Geometry: final body of the model. Coordinates: model frame, mm. A direction names the side the tool comes from. Give positions to 0.01 mm unless a question says otherwise; leave off trailing zeros. Loops run counter-clockwise (first coordinate to the right, second up) from the corner with the lowest first, then second, coordinate; pieces in that order, holes last.
Autodesk Inventor part; units mm, degrees
ref_plane "Work Plane1" through (-26, 27.7, 10) normal (0, -1, 0) x (1, 0, 0)
ref_plane "Work Plane3" through (19.5, 27.7, -10) normal (0, -1, 0) x (1, 0, 0)
ref_plane "Work Plane5" through (-19.5, 27.7, 10) normal (0, 0, 1) x (1, 0, 0)
ref_plane "Work Plane1" through (-26, 27.7, 10) normal (0, -1, 0) x (1, 0, 0)
sketch "Sketch1" plane through (-26, 27.7, 10) normal (0, -1, 0) x (1, 0, 0)
  line L0 (6, -0.5) -> (6, 0)
  line L1 (0, 0) -> (6.5, 0)
  line L2 (6, 0) -> (0, 0)
  line L3 (0, 0) -> (-2, 0)
  arc A0 (0, 0) -> (-2, -2) centre (0, -2) ccw
  line L4 (-2, 0) -> (-2, 0)
  line L5 (0, 0) -> (-2, 0)
  line L6 (-2, -2) -> (-2, -3.75)
  line L7 (-2, -2) -> (-2, 0)
  arc A1 (0, 0) -> (-2, -2) centre (0, -2) ccw
  line L8 (0, 0) -> (-2, 0)
  arc A2 (-2, -18) -> (0, -20) centre (0, -18) ccw
  line L9 (-2, -2) -> (-2, -18)
  line L10 (-2, -18) -> (-2, -20)
  line L11 (-2, -20) -> (0, -20)
  line L12 (0, -20) -> (6.5, -20)
  line L13 (6, -19.5) -> (6, -20)
  line L14 (6, -19.5) -> (6, -0.5)
  point P0 (26, -10)
extrude "Extrusion1" add sketch "Sketch1" along normal blind 10
ref_plane "Work Plane3" through (19.5, 27.7, -10) normal (0, -1, 0) x (1, 0, 0)
sketch "Sketch2" plane through (19.5, 27.7, -10) normal (0, -1, 0) x (1, 0, 0)
  line L0 (0.5, 19.5) -> (0.5, 0.5)
  line L1 (0.5, 19.5) -> (0.5, 20)
  line L2 (0, 20) -> (6.5, 20)
  line L3 (0.5, 0.4979) -> (0.5, -0.0021)
  arc A0 (6.5, 0) -> (8.5, 2) centre (6.5, 2) ccw
  line L4 (0, 0) -> (6.5, 0)
  line L5 (8.5, 2) -> (6.5, 2)
  line L6 (6.5, 2) -> (6.5, 0)
  line L7 (6.5, 0) -> (8.5, 0)
  line L8 (8.5, 0) -> (8.5, 2)
  line L9 (0.5, 20) -> (8.5, 20)
  line L10 (8.5, 20) -> (8.5, 0)
  line L11 (8.5, 0) -> (0.5, 0)
  line L12 (0.5, 0) -> (0.5, 20)
  point P0 (-19.5, 10)
  point P1 (0.5, 0.5)
  dimension "d4" = 0.5
extrude "Extrusion2" add sketch "Sketch2" along normal blind 10
ref_plane "Work Plane5" through (-19.5, 27.7, 10) normal (0, 0, 1) x (1, 0, 0)
sketch "Sketch3" plane through (-19.5, 27.7, 10) normal (0, 0, 1) x (1, 0, 0)
  line L0 (-8.5, 0) -> (-8.5, -10)
  line L1 (47.5, 0) -> (47.5, 2.5)
  line L2 (-8.5, -10) -> (47.5, -10)
  line L3 (47.5, -10) -> (47.5, 2.5)
  line L4 (47.5, 2.5) -> (-8.5, 2.5)
  line L5 (-8.5, 2.5) -> (-8.5, -10)
  point P0 (19.5, -27.7)
extrude "Extrusion3" add sketch "Sketch3" along normal blind 10
ref_plane "Work Plane4" through (19.5, 27.7, -10) normal (0, 1, 0) x (1, 0, 0)
sketch "Sketch4" plane through (19.5, 27.7, -10) normal (0, 1, 0) x (1, 0, 0)
  arc A0 (6.415, -13.3929) -> (6.415, -16.6071) centre (4.5, -15) ccw
  circle A1 centre (4.5, -15) radius 2.5
  arc A2 (6.415, -3.3929) -> (6.415, -6.6071) centre (4.5, -5) ccw
  circle A3 centre (4.5, -5) radius 2.5
  arc A4 (-45.415, -16.6071) -> (-45.415, -13.3929) centre (-43.5, -15) ccw
  circle A5 centre (-43.5, -15) radius 2.5
  arc A6 (-45.415, -6.6071) -> (-45.415, -3.3929) centre (-43.5, -5) ccw
  circle A7 centre (-43.5, -5) radius 2.5
  point P0 (-19.5, -10)
  point P1 (6.415, -3.3929)
  point P2 (6.415, -13.3929)
  point P3 (-45.415, -16.6071)
  point P4 (-45.415, -6.6071)
extrude "Extrusion4" cut sketch "Sketch4" against normal blind 10
ref_plane "Work Plane6" through (-28, 30.2, -3.75) normal (-1, 0, 0) x (0, 0, 1)
sketch "Sketch5" plane through (-28, 30.2, -3.75) normal (-1, 0, 0) x (0, 0, 1)
  line L0 (-6.25, -12.5) -> (23.75, -12.5)
  line L1 (-6.25, -2.5) -> (-6.25, -12.5)
  line L2 (23.75, -12.5) -> (-6.25, -12.5)
  line L3 (-6.25, -12.5) -> (-6.25, -2.5)
  line L4 (-6.25, -2.5) -> (23.75, -2.5)
  line L5 (23.75, -2.5) -> (23.75, -12.5)
  point P0 (3.75, -30.2)
extrude "Extrusion5" add sketch "Sketch5" along normal blind 11.915
ref_plane "Work Plane7" through (19.5, 27.7, -10) normal (0, 0, -1) x (-1, 0, 0)
sketch "Sketch6" plane through (19.5, 27.7, -10) normal (0, 0, -1) x (-1, 0, 0)
  line L0 (39.5, 0) -> (39.5, -10)
  line L1 (47.5, 0) -> (59.415, 0)
  line L2 (39.5, -10) -> (59.415, -10)
  line L3 (59.415, -10) -> (59.415, 0)
  line L4 (59.415, 0) -> (39.5, 0)
  line L5 (39.5, 0) -> (39.5, -10)
  point P0 (19.5, -27.7)
extrude "Extrusion6" add sketch "Sketch6" along normal blind 10
ref_plane "Work Plane8" through (-39.915, 30.2, -3.75) normal (-1, 0, 0) x (0, 0, 1)
sketch "Sketch7" plane through (-39.915, 30.2, -3.75) normal (-1, 0, 0) x (0, 0, 1)
  line L0 (-16.25, -12.5) -> (-16.25, -2.5)
  line L1 (-16.25, -12.5) -> (-6.25, -12.5)
  line L2 (-6.25, -12.5) -> (-6.25, -2.5)
  line L3 (-6.25, -2.5) -> (-16.25, -2.5)
  line L4 (-16.25, -2.5) -> (-16.25, -12.5)
  line L5 (23.75, -12.5) -> (23.75, -2.5)
  line L6 (23.75, -2.5) -> (13.75, -2.5)
  line L7 (13.75, -2.5) -> (13.75, -12.5)
  line L8 (13.75, -12.5) -> (23.75, -12.5)
  line L9 (23.75, -12.5) -> (23.75, -2.5)
  point P0 (3.75, -30.2)
  point P1 (23.75, -12.5)
  dimension "d15" = 10
  dimension "d16" = 10
extrude "Extrusion7" add sketch "Sketch7" along normal blind 20
ref_plane "Work Plane9" through (19.5, 27.7, -20) normal (0, 0, -1) x (-1, 0, 0)
sketch "Sketch9" plane through (-26, 17.7, 10) normal (0, -1, 0) x (1, 0, 0)
  line L0 (-13.915, 0) -> (-33.915, 0)
  line L1 (-13.915, 0) -> (-33.915, 0)
  line L2 (-33.915, 0) -> (-33.915, 10)
  line L3 (-33.915, 10) -> (-13.915, 10)
  line L4 (-13.915, 10) -> (-13.915, 0)
  point P0 (26, -10)
  point P1 (-33.915, 0)
extrude "Extrusion9" add sketch "Sketch9" along normal blind 20
ref_plane "Work Plane2" through (-39.915, 27.7, 15) normal (0, 0, -1) x (-1, 0, 0)
sketch "Sketch10" plane through (-39.915, 27.7, 15) normal (0, 0, -1) x (-1, 0, 0)
  line L0 (20, -30) -> (0, -30)
  line L1 (-59.915, -10) -> (-67.915, -10)
  line L2 (0, -30) -> (-59.915, -10)
  line L3 (0, -30) -> (0, -10)
  line L4 (0, -10) -> (-59.915, -10)
  point P0 (-39.915, -27.7)
extrude "Extrusion10" add sketch "Sketch10" along normal mid plane 4
ref_plane "Work Plane10" through (-19.5, 27.7, 20) normal (0, 0, 1) x (1, 0, 0)
thread "Thread1"
thread "Thread2"
thread "Thread3"
thread "Thread4"
sketch "Sketch13" plane through (-19.5, 27.7, 20) normal (0, 0, 1) x (1, 0, 0)
  line L0 (-20.415, -10) -> (-20.415, 0)
  line L1 (-20.415, 0) -> (-30.415, 0)
  line L2 (-20.415, 0) -> (-40.415, 0)
  line L3 (-30.415, 0) -> (-30.415, -5)
  line L4 (-20.415, -10) -> (-20.415, -30)
  line L5 (-20.415, -30) -> (-20.415, -20)
  line L6 (-20.415, -20) -> (-30.415, -20)
  circle A0 centre (-30.415, -5) radius 2.5
  circle A1 centre (-30.415, -20) radius 2.5
  point P0 (19.5, -27.7)
  dimension "d40" = 10
  dimension "d41" = 5
  dimension "d42" = 10
  dimension "d43" = 10
  dimension "d44" = 5
  dimension "d45" = 5
extrude "Extrusion12" cut sketch "Sketch13" against normal through all
sketch "Sketch14" plane through (-59.915, 27.7, -10) normal (0, 0, 1) x (1, 0, 0)
  line L0 (20, 0) -> (20, -10)
  line L1 (0, -10) -> (0, 0)
  line L2 (20, 0) -> (0, 0)
  line L3 (0, 0) -> (0, -10)
  line L4 (0, -10) -> (20, -10)
  line L5 (20, -10) -> (20, 0)
  point P0 (59.915, -27.7)
  point P1 (20, -10)
extrude "Extrusion13" add sketch "Sketch14" against normal blind 2
sketch "Sketch15" plane through (-39.915, 27.7, 10) normal (0, 0, -1) x (-1, 0, 0)
  line L0 (20, -30) -> (0, -30)
  line L1 (20, 0) -> (0, 0)
  line L2 (0, 0) -> (0, -30)
  line L3 (0, -30) -> (20, -30)
  line L4 (20, -30) -> (20, 0)
  point P0 (-39.915, -27.7)
extrude "Extrusion14" cut sketch "Sketch15" against normal blind 2
sketch "Sketch16" plane through (-39.915, 27.7, 12) normal (0, 0, -1) x (-1, 0, 0)
  line L0 (-11.915, 0) -> (20, 0)
  line L1 (20, -30) -> (0, -30)
  line L2 (20, 0) -> (0, 0)
  line L3 (0, 0) -> (0, -30)
  line L4 (0, -30) -> (20, -30)
  line L5 (20, -30) -> (20, 0)
  circle A0 centre (10, -20) radius 2.5
  circle A1 centre (10, -20) radius 2.5
  circle A2 centre (10, -5) radius 2.5
  circle A3 centre (10, -5) radius 2.5
  point P0 (-39.915, -27.7)
  point P1 (0, 0)
extrude "Extrusion15" add sketch "Sketch16" along normal blind 4
sketch "Sketch17" plane through (-49.915, 22.7, -12) normal (0, 0, -1) x (-1, 0, 0)
  circle A0 centre (0, 0) radius 2.5
  point P0 (-49.915, -22.7)
extrude "Extrusion16" cut sketch "Sketch17" against normal blind 4
sketch "Sketch18" plane through (-59.915, 27.7, -10) normal (0, 0, 1) x (1, 0, 0)
  line L0 (0, -10) -> (0, 0)
  line L1 (20, 0) -> (0, 0)
  line L2 (0, -10) -> (20, -10)
  line L3 (20, -10) -> (20, 0)
  line L4 (20, 0) -> (0, 0)
  line L5 (0, 0) -> (0, -10)
  point P0 (59.915, -27.7)
extrude "Extrusion17" cut sketch "Sketch18" against normal blind 2
properties part number "servo_holder" material "PET Plastic"
Item 1: Section query A-A on y = 22.7. Return loops of the section in (x, z) (3 decimals).
Values follow:
outline: (-59.915, -20) - (-52.415, -20) - (-52.415, -12) - (-59.915, -12) - close; (-59.915, 8) - (-52.415, 8) - (-52.415, 20) - (-59.915, 20) - close; (-47.415, -20) - (-20, -20) - (-20, 10) - (20, 10) - (20, -10) - (28, -10) - (28, 20) - (-47.415, 20) - (-47.415, 8) - (-39.915, 8) - (-39.915, -12) - (-47.415, -12) - close; hole circle Ø5 at (-24, -5); hole circle Ø5 at (-24, 5); hole circle Ø5 at (24, -5); hole circle Ø5 at (24, 5)
Item 2: Section query B-B on z = -5. Return loops of the section in (x, y) (3 decimals).
Values follow:
outline: (-39.915, 17.7) - (-26.5, 17.7) - (-26.5, 27.7) - (-39.915, 27.7) - close; (-21.5, 17.7) - (-20, 17.7) - (-20, 27.7) - (-21.5, 27.7) - close; (20, 17.7) - (21.5, 17.7) - (21.5, 27.7) - (20, 27.7) - close; (26.5, 17.7) - (28, 17.7) - (28, 27.7) - (26.5, 27.7) - close
Item 3: Section query C-C on x = 24. Return loops of the section in (y, z).
Values follow:
outline: (17.7, -10) - (27.7, -10) - (27.7, -7.5) - (17.7, -7.5) - close; (17.7, -2.5) - (27.7, -2.5) - (27.7, 2.5) - (17.7, 2.5) - close; (17.7, 7.5) - (27.7, 7.5) - (27.7, 10) - (30.2, 10) - (30.2, 20) - (17.7, 20) - close
Item 4: Section query D-D on z = 14. Return loops of the section in (x, y) (3 decimals).
Values follow:
outline: (-59.915, -2.3) - (-39.915, -2.3) - (20, 17.7) - (28, 17.7) - (28, 30.2) - (-28, 30.2) - (-28, 27.7) - (-59.915, 27.7) - close; hole circle Ø5 at (-49.915, 7.7); hole circle Ø5 at (-49.915, 22.7)
Item 5: Pin query (flat end, axial travel): pin 1 (5 mm diameter, centred on x = -42, y = 14, fed in from -Z); pin 2 (8 mm diameter, centred on x = -38.5, z = 6, fed in from -Y); pin 3 (4 mm diameter, centred on x = 25, y = 25, fed in from -Z); pin 4 (16 mm diameter, centred on x = -11, y = 3, fed in from -Z). Return the tip coordinate at first contact, or that it passes through.
Values follow:
pin 1: stops at z = 8
pin 2: stops at y = -2.3
pin 3: stops at z = -10
pin 4: stops at z = 13
Item 6: Draft query along X for faces 1 (the face through (28, 22, 5)), 2 (the face through (0, 24, 10)), 3 (the face through (-52.3, 23.9, -12)). Return one class per face: +X half, -X half, draft (parallel to the pull), parting line (faces both ways), or undercut.
Values follow:
face 1: +X half
face 2: undercut
face 3: draft
Item 7: Ray query, probe 1 along Z at (x, y) = (24, 24); probe 2 along X at (y, z) = (22.7, 10.15) (3 decimals); probe 3 along X at (y, z) = (21.75, -5) (3 decimals). Return the intervals inside material, ascending.
Values follow:
probe 1: z = -10 to -7.5, -2.5 to 2.5, 7.5 to 20
probe 2: x = -59.915 to -52.415, -47.415 to 28
probe 3: x = -39.915 to -26.5, -21.5 to -20, 20 to 21.5, 26.5 to 28
Item 8: Set-up query: faces 4 (the face through (24, 23, -10)), 5 (the face through (20, 23, 0)), 6 (the face through (-39.915, 8, 19)), 7 (the face through (-28, 29, 15)). Return all of +Z, -Z, +X, -X, +Y, -Y with unobstructed straight access to the full face (end or side cutting, diameter ignored); none if empty.
Values follow:
face 4: -Z, +X, +Y, -Y
face 5: -Z, +Y, -Y
face 6: +Z, +X, -Y
face 7: +Z, -Z, -X, +Y
